from build123d import *

# Parameters (mm, degrees)
SKETCH1_R               = 21
BOSS_EXTRUDE1_DEPTH     = 3
CHAMFER1_SIZE           = 2
FILLET1_R               = 0.1
SKETCH2_R               = 21
BOSS_EXTRUDE2_DEPTH     = 12
FILLET2_R               = 0.1
SKETCH3_R               = 21
BOSS_EXTRUDE3_DEPTH     = 6
SKETCH4_R               = 3
SKETCH4_R_2             = 1.5
CUT_EXTRUDE1_DEPTH      = 6
BOSS_EXTRUDE4_DEPTH     = 6
CHAMFER2_SIZE           = 1
CUT_EXTRUDE2_DEPTH      = 55.134670037
CUT_EXTRUDE2_DEPTH_BACK = 55.134670037
SKETCH6_R               = 1.5
BOSS_EXTRUDE5_DEPTH     = 1
SKETCH8_R               = 2.25
BOSS_EXTRUDE6_DEPTH     = 4
SKETCH9_R               = 1.25
CUT_EXTRUDE3_DEPTH      = 4
SKETCH10_W              = 3.229244049
SKETCH10_H              = 6.822780719
SKETCH10_H_2            = 3.229244049
BOSS_EXTRUDE7_DEPTH     = 8


with BuildPart() as part:
    # Sketch1 → Boss-Extrude1 (new body)
    with BuildSketch(Plane.XY):
        Circle(SKETCH1_R)
    extrude(amount=BOSS_EXTRUDE1_DEPTH)

    # Chamfer1
    chamfer1_edges = [part.edges().sort_by_distance(p)[0] for p in [
        (-21, 0, 0),
    ]]
    chamfer(chamfer1_edges, length=CHAMFER1_SIZE)

    # Fillet1
    fillet1_edges = [part.edges().sort_by_distance(p)[0] for p in [
        (-21, 0, 3),
    ]]
    fillet(fillet1_edges, radius=FILLET1_R)

    # Sketch2 → Boss-Extrude2 (add)
    with BuildSketch(Plane.XY.offset(3)):
        Circle(SKETCH2_R)
    extrude(amount=BOSS_EXTRUDE2_DEPTH)

    # Fillet2
    fillet2_edges = [part.edges().sort_by_distance(p)[0] for p in [
        (-21, 0, 15),
    ]]
    fillet(fillet2_edges, radius=FILLET2_R)

    # Sketch3 → Boss-Extrude3 (add)
    with BuildSketch(Plane.XY.offset(15)):
        Circle(SKETCH3_R)
    extrude(amount=BOSS_EXTRUDE3_DEPTH)

    # Sketch4 → Cut-Extrude1 (cut)
    with BuildSketch(Plane(origin=(0, 0, 0), x_dir=(-1, 0, 0), z_dir=(0, 0, -1))):
        Circle(SKETCH4_R)
        with Locations((-10, 0)):
            Circle(SKETCH4_R_2)
        with Locations((0, 10)):
            Circle(SKETCH4_R_2)
        with Locations((10, 0)):
            Circle(SKETCH4_R_2)
        with Locations((0, -10)):
            Circle(SKETCH4_R_2)
    extrude(amount=-CUT_EXTRUDE1_DEPTH, mode=Mode.SUBTRACT)

    # Sketch5 → Boss-Extrude4 (add)
    with BuildSketch(Plane.XY.offset(17)):
        with BuildLine():
            Line((21.633307653, -11.5), (33.25, -11.5))
            Line((33.25, -11.5), (33.25, -15.5))
            Line((33.25, -15.5), (-33.25, -15.5))
            Line((-33.25, -15.5), (-33.25, -11.5))
            Line((-33.25, -11.5), (-21.633307653, -11.5))
            ThreePointArc((-21.633307653, -11.5), (0, 24.5), (21.633307653, -11.5))
        make_face()
    extrude(amount=BOSS_EXTRUDE4_DEPTH)

    # Chamfer2
    chamfer2_edges = [part.edges().sort_by_distance(p)[0] for p in [
        (0, 24.5, 17),
        (-27.441653826, -11.5, 17),
        (-33.25, -13.5, 17),
        (33.25, -13.5, 17),
        (27.441653826, -11.5, 17),
        (0, 24.5, 23),
        (-27.441653826, -11.5, 23),
        (-33.25, -13.5, 23),
        (33.25, -13.5, 23),
        (27.441653826, -11.5, 23),
    ]]
    chamfer(chamfer2_edges, length=CHAMFER2_SIZE)

    # Sketch6 → Cut-Extrude2 (cut, two sides: drawn at the far end of the back side and taken through both)
    with BuildSketch(Plane(origin=(0, -11.5, 0), x_dir=(1, 0, 0), z_dir=(0, 1, 0)).offset(-CUT_EXTRUDE2_DEPTH_BACK)):
        with Locations(Location((-28.5, -20, 0), (0, 0, 180))):
            Circle(SKETCH6_R)
        with Locations(Location((28.5, -20, 0), (0, 0, 180))):
            Circle(SKETCH6_R)
    extrude(amount=CUT_EXTRUDE2_DEPTH + CUT_EXTRUDE2_DEPTH_BACK, mode=Mode.SUBTRACT)

    # Sketch7 → Boss-Extrude5 (add)
    with BuildSketch(Plane.XY.offset(23)):
        with BuildLine():
            Line((12.499599994, -16.5), (-12.499599994, -16.5))
            ThreePointArc((-12.499599994, -16.5), (0, 20.7), (12.499599994, -16.5))
        make_face()
    extrude(amount=BOSS_EXTRUDE5_DEPTH)

    # Sketch8 → Boss-Extrude6 (add)
    with BuildSketch(Plane.XY.offset(24)):
        with Locations((-12.5, 12.5)):
            Circle(SKETCH8_R)
        with Locations((12.5, 12.5)):
            Circle(SKETCH8_R)
        with Locations((12.5, -12.5)):
            Circle(SKETCH8_R)
        with Locations((-12.5, -12.5)):
            Circle(SKETCH8_R)
    extrude(amount=BOSS_EXTRUDE6_DEPTH)

    # Sketch9 → Cut-Extrude3 (cut)
    with BuildSketch(Plane.XY.offset(28)):
        with Locations((12.5, 12.5)):
            Circle(SKETCH9_R)
        with Locations((12.5, -12.5)):
            Circle(SKETCH9_R)
        with Locations((-12.5, 12.5)):
            Circle(SKETCH9_R)
        with Locations((-12.5, -12.5)):
            Circle(SKETCH9_R)
    extrude(amount=-CUT_EXTRUDE3_DEPTH, mode=Mode.SUBTRACT)

    # Sketch10 → Boss-Extrude7 (add)
    with BuildSketch(Plane.XY.offset(24)):
        with Locations((16.831288736, 2.056395103)):
            Rectangle(SKETCH10_W, SKETCH10_H)
        with Locations((16.831288736, -5.561216158)):
            Rectangle(SKETCH10_W, SKETCH10_H_2)
    extrude(amount=BOSS_EXTRUDE7_DEPTH)


solid = part.part
Input: part model. Units: mm. Frame: model coordinates. A direction names the side the tool comes from. Round coordinates to 2 decimals unless told otherwise and drop trailing zeros. Loops run counter-clockwise (first coordinate to the right, second up) from the corner with the lowest first, then second, coordinate; pieces in that order, holes last. Notation, with made-up numbers: M -20.5,-29 L 8.5,-29 A22 cw 8.5,-3 Z; hole C 25,51.25 d10. An arc over 180 degrees is marked long. Answer as CSV lines item,"result". Start each with the question number.
(1) Draft query along Y for faces 1 (the cylindrical face through (-8.5, 0.07, 2.96)), 2 (the cylindrical face through (20.03, 6.31, 2.44)), 3 (the flat face through (17, -3.947, 28)), 4 (the flat face through (15.217, -6, 28)). Return one class per face: released by +Y, released by -Y, zero draft, split by the parting line, or undercut.
(2) Section D-D, the plane z = 12.5. Output: boundary loops of the cut face in (x, y), plus the area to 3 significant figures.
(3) First-contact query: pin 1 (12 mm diameter, centred on x = -6.5, z = 5, fed in from -Y); pin 2 (4 mm diameter, centred on x = 5.5, z = 23.5, fed in from -Y); pin 3 (3.5 mm diameter, centred on x = 16.5, z = 29, fed in from -Y). Flat tips, straight axial feed; report the tip coordinate or a pass-through.
(4) Section C-C, the plane z = 20. Output: boundary loops of the cut face in (x, y).
(5) Section B-B, the plane x = -28.5. Output: boundary loops of the cut face in (y, z).
(6) Reachability of faces 5 (the flat face through (18.446, -6, 28)), 6 (the flat face through (-26, -11.5, 20)), 7 (the flat face through (0, 0, 6)) from +Z, -Z, +X, -X, +Y, -Y: full face, straight path, thin tool, end or side. Return the list, or none.
(7) Section A-A, the plane z = 25. State how many separate pieces and enclosed holes the cut face has, plus the area to 3 significant figures.
Values found:
1,face 1,"undercut"
1,face 2,"split by the parting line"
1,face 3,"undercut"
1,face 4,"zero draft"
2,outline,"C 0,0 d42"
2,area,"1,390 mm²"
3,pin 1,"stops at y = -20.99"
3,pin 2,"stops at y = -16.5"
3,pin 3,"stops at y = -7.18"
4,outline,"M -33.25,-15.5 L -30,-15.5 L -30,-11.5 L -33.25,-11.5 Z; M -27,-15.5 L -14.17,-15.5 A21 ccw 14.17,-15.5 L 27,-15.5 L 27,-11.5 L 21.63,-11.5 A24.5 ccw long -21.63,-11.5 L -27,-11.5 Z; M 30,-15.5 L 33.25,-15.5 L 33.25,-11.5 L 30,-11.5 Z"
5,outline,"M -15.5,17 L -12.5,17 L -11.5,18 L -11.5,18.5 L -15.5,18.5 Z; M -15.5,21.5 L -11.5,21.5 L -11.5,22 L -12.5,23 L -15.5,23 Z"
6,face 5,"+Z, +X, +Y, -Y"
6,face 6,"+Z, -Z, -X"
6,face 7,"-Z"
7,separate pieces,"6"
7,enclosed holes,"4"
7,area,"76.4 mm²"
